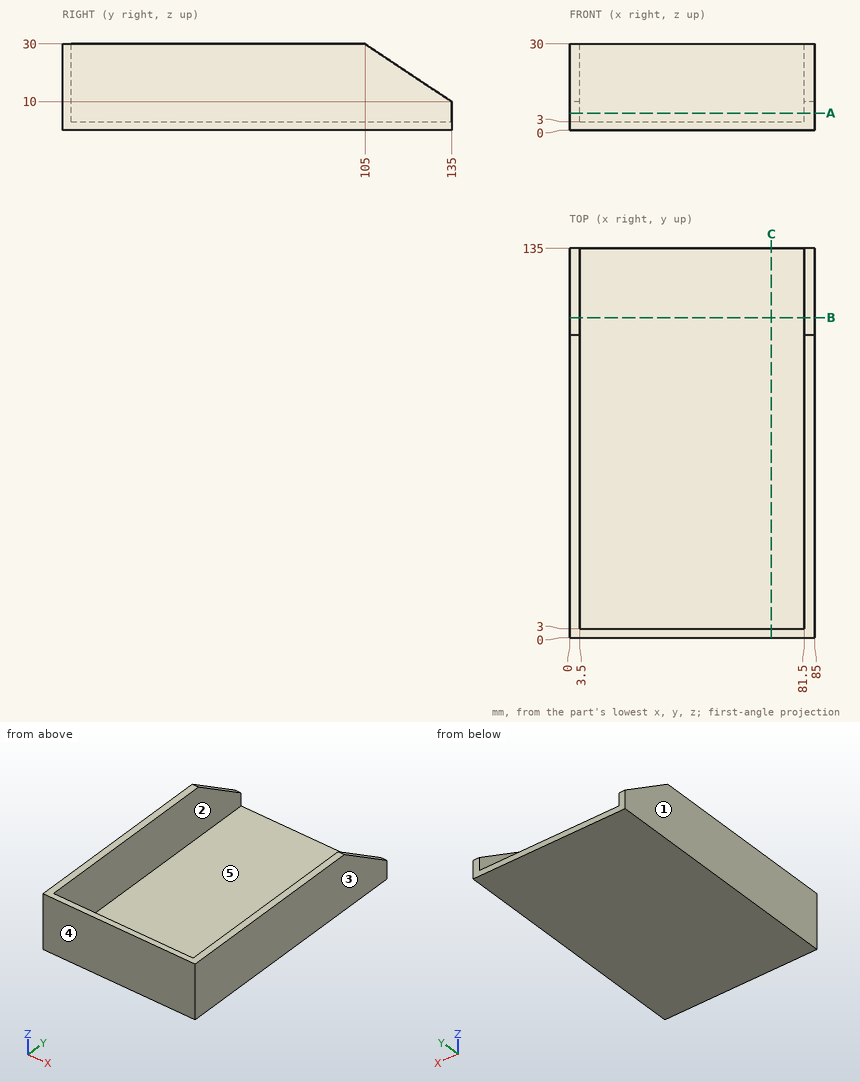
Can you work these out from the drawing? Everything is in mm from the part's minimum corner. A direction names the side the tool comes from. Coordinates: 2 decimals unless noted, no trailing zeros. Loops run counter-clockwise (first coordinate to the right, second up) from the corner with the lowest first, then second, coordinate; pieces in that order, holes last. Notation, with made-up numbers: M 14.5,-36 L 19.5,-36 A30 ccw 19.5,-5 Z; hole C 7.5,67.25 d7. An arc over 180 degrees is marked long. One line per item, written item: value.
1. Thinking about a two-plate mould opening in X: for the marked faces 1, 2 and 3, which applies, +X half, -X half, draft (parallel to the pull), parting line (faces both ways), or undercut?
Geometry says:
face 1: -X half
face 2: undercut
face 3: +X half
2. Please list where these lines run through material, in increasing order: probe 1 along X at (y, z) = (80, 28.5); probe 2 along Y at (x, z) = (65.5, 14.5).
Geometry says:
probe 1: x = 0 to 3.5, 81.5 to 85
probe 2: y = 0 to 3
3. On a 3-axis mill with a long thin cutter (end or side, diameter ignored), from which of +Z, -Z, +X, -X, +Y, -Y can I reach the whole of each face in a straight line? I mean the marked faces 4 and 5. Say none if no direction works.
Geometry says:
face 4: +Z, -Z, +X, -X, -Y
face 5: +Z, +Y
4. Imagine slicing it at A-A (z = 6). List the corners of the cut face in (x, y) for me.
Geometry says:
outline: M 0,0 L 85,0 L 85,135 L 81.5,135 L 81.5,3 L 3.5,3 L 3.5,135 L 0,135 Z
5. Will this pin go through, and if not, where does the flat tip stop? pin 1 Ø6 at (x, y) = (9, 64) entering from +Z.
Geometry says:
pin 1: stops at z = 3
6. Imagine slicing it at B-B (y = 111). List the corners of the cut face in (x, z) for me.
Geometry says:
outline: M 0,0 L 85,0 L 85,26 L 81.5,26 L 81.5,3 L 3.5,3 L 3.5,26 L 0,26 Z
7. Imagine slicing it at C-C (x = 70). List the corners of the cut face in (y, z) for me, and give its area (3 significant figures).
Geometry says:
outline: M 0,0 L 135,0 L 135,3 L 3,3 L 3,30 L 0,30 Z
area: 486 mm2
